```python
from build123d import *

# Parameters (mm, degrees)
SKETCH2_R                               = 140
BOSS_EXTRUDE1_DEPTH                     = 12
SKETCH3_R                               = 16
SKETCH3_R_2                             = 8.5
CUT_EXTRUDE1_DEPTH                      = 13
CBORE_FOR_M5_HEX_HEAD_BOLT1_D           = 9
CBORE_FOR_M5_HEX_HEAD_BOLT1_CBORE_D     = 16
CBORE_FOR_M5_HEX_HEAD_BOLT1_CBORE_DEPTH = 7


with BuildPart() as part:
    # Sketch2 → Boss-Extrude1 (new body)
    with BuildSketch(Plane.XY):
        Circle(SKETCH2_R)
    extrude(amount=BOSS_EXTRUDE1_DEPTH)

    # Sketch3 → Cut-Extrude1 (cut, through all)
    with BuildSketch(Plane.XY.offset(12)):
        with Locations((59.451586038, 53.530448509)):
            Circle(SKETCH3_R)
        with Locations((0, 80)):
            Circle(SKETCH3_R)
        with Locations((79.561751629, -8.362277061)):
            Circle(SKETCH3_R)
        with Locations((47.022820183, -64.72135955)):
            Circle(SKETCH3_R)
        with Locations((4.186876499, -79.89036278)):
            Circle(SKETCH3_R_2)
        with Locations((-36.319239979, -71.280521935)):
            Circle(SKETCH3_R_2)
        with Locations((-67.093645436, -43.571122801)):
            Circle(SKETCH3_R_2)
        with Locations((-79.89036278, -4.186876499)):
            Circle(SKETCH3_R_2)
        with Locations((-71.280521935, 36.319239979)):
            Circle(SKETCH3_R_2)
        with Locations((-43.571122801, 67.093645436)):
            Circle(SKETCH3_R_2)
    extrude(amount=-CUT_EXTRUDE1_DEPTH, mode=Mode.SUBTRACT)

    # CBORE for M5 Hex Head Bolt1 (through all)
    with Locations(Plane.XY.offset(12)):
        with Locations((0, 0)):
            CounterBoreHole(CBORE_FOR_M5_HEX_HEAD_BOLT1_D / 2, CBORE_FOR_M5_HEX_HEAD_BOLT1_CBORE_D / 2, CBORE_FOR_M5_HEX_HEAD_BOLT1_CBORE_DEPTH)


solid = part.part
```
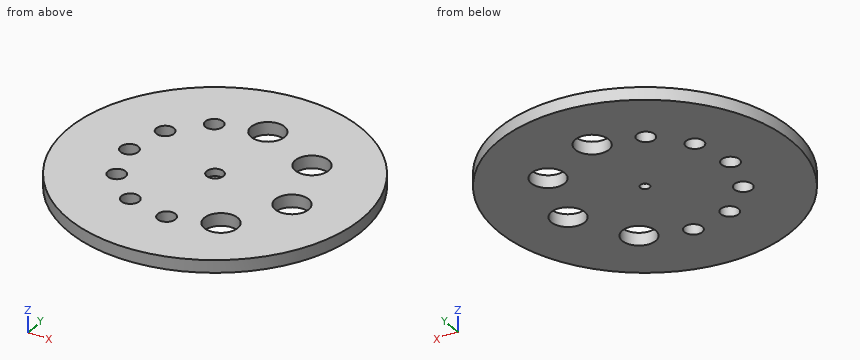
Design review of the part built by this model. Coordinates are the model's own, in mm. Give positions to 0.01 mm unless a question says otherwise; leave off trailing zeros. Order: outer loops, then holes, each group sorted by start corner. A loop starts at its lowest first (then second) coordinate and runs counter-clockwise, first axis right, second up. Notation, with made-up numbers: (37, 25.5) - (77, 25.5) arc R30 cw to (77, 60.5) - close; hole circle Ø8 at (30.25, -36.5). An arc over 180 degrees is marked (long way). Use a Markdown table: item, result. Add a question column.
(1) Wall thickness on probe 1 along Y at (x, z) = (-71, 10); probe 2 along X at (y, z) = (41, 6.25); probe 3 along X at (y, z) = (-75, 7.5): over which ranges is each line inside the solid? List them lowest first. Write a range as [from, to].
(2) Clearance check with flat-ended pins moving along their axes: P1, Ø13.5, axis at x = -71.28, y = 36.32, coming from the +Z side; P2, Ø2, axis at y = 96.5, z = 7.5, coming from the +X side; P3, Ø3, axis at x = 94, z = 2.5, coming from the +Y side; P4, Ø4, axis at y = 6, z = 2.5, coming from the +X side. State where each tip first meets the part, or that it passes through.
(3) Add section B-B on y = -76.5. Give the boundary of the cut face in (x, z), then the cut area to 3 significant figures.
(4) Add section D-D on z = 9. Give the number of separate pieces and of enclosed holes in the cut face, then the cut area to 3 significant figures.
(5) Add section A-A on x = 0. Give the boundary of the cut face in (y, z).
(6) Add section C-C on x = 57. Give the boundary of the cut face in (y, z).
Report:
| question | item | result |
|---|---|---|
| 1 | probe 1 | y = [-120.66, -51.12], [-36.02, 27.82], [44.81, 120.66] |
| 1 | probe 2 | x = [-133.86, -78.38], [-64.19, 49.5], [69.4, 133.86] |
| 1 | probe 3 | x = [-118.22, -43.96], [-28.68, -2.77], [11.14, 34.76], [59.28, 118.22] |
| 2 | P1 | passes through |
| 2 | P2 | stops at x = 102.37 |
| 2 | P3 | stops at y = 105.09 |
| 2 | P4 | stops at x = 139.94 |
| 3 | outline | (-117.25, 0) - (-43.03, 0) - (-43.03, 12) - (-117.25, 12) - close; (-29.61, 0) - (-3.61, 0) - (-3.61, 12) - (-29.61, 12) - close; (11.98, 0) - (36.19, 0) - (36.19, 12) - (11.98, 12) - close; (57.85, 0) - (117.25, 0) - (117.25, 12) - (57.85, 12) - close |
| 3 | area | 2,210 mm² |
| 4 | separate pieces | 1 |
| 4 | enclosed holes | 11 |
| 4 | area | 56,800 mm² |
| 5 | outline | (-140, 0) - (-87.29, 0) - (-87.29, 12) - (-140, 12) - close; (-72.49, 0) - (-4.5, 0) - (-4.5, 5) - (-8, 5) - (-8, 12) - (-72.49, 12) - close; (4.5, 0) - (64, 0) - (64, 12) - (8, 12) - (8, 5) - (4.5, 5) - close; (96, 0) - (140, 0) - (140, 12) - (96, 12) - close |
| 6 | outline | (-127.87, 0) - (-77.23, 0) - (-77.23, 12) - (-127.87, 12) - close; (-52.21, 0) - (37.72, 0) - (37.72, 12) - (-52.21, 12) - close; (69.34, 0) - (127.87, 0) - (127.87, 12) - (69.34, 12) - close |
